Geometry check sheet. Reference: the model listing, model coordinates, mm. Round coordinates to 2 decimals unless told otherwise and drop trailing zeros. Write each loop counter-clockwise with the first axis right and the second up, starting at its lowest first coordinate (ties: lowest second). Pieces come first, ordered by that corner, then holes.
Item 1: Depth check by flat-ended pin: P1, Ø6.5, axis at x = -259.97, y = -86.86, coming from the -Z side; P2, Ø2, axis at y = -197.5, z = -4, coming from the -X side; P3, Ø2, axis at y = 218, z = -1, coming from the +X side. Enter the tip coordinate at first touch or a pass-through.
Item 2: Cross-section at A-A (z = -2.5). Enter the section's corners in (x, y).
Item 3: Draft check along X on faces 1 (the face through (288.249, 120.906, -5.706)), 2 (the face through (-28, 27, 0)). Enter one of: pulls with the +X half, pulls with the -X half, needs draft (parallel to the pull), parting line crosses it, or undercut.
Item 4: Scan lines: probe 1 along Y at (x, z) = (174.5, -4); probe 2 along X at (y, z) = (16, -5.5); probe 3 along X at (y, z) = (157, -2.5). Record each from-to range of solid material in increasing order.
from build123d import *

# Parameters (mm, degrees)
F0_R     = 327.025
F1_DEPTH = 6.35
F3_D     = 7.9375
F5_D     = 7.9375
F6_R     = 5.08


with BuildPart() as f1:
    # F0 (on Top) → F1 (new body)
    with BuildSketch(Plane.XY):
        with Locations((-23.674974, 22.676632)):
            Circle(F0_R)
    extrude(amount=-F1_DEPTH)

    # F3 (through all)
    with Locations(Plane.XY):
        with Locations((-259.972523, 22.676632), (209.927477, 22.676632)):
            Hole(F3_D / 2)

    # F5 (through all)
    with Locations(Plane.XY):
        with Locations((-259.972523, 132.214132), (-259.972523, -86.860868), (209.927477, -86.860868), (209.927477, 132.214132)):
            Hole(F5_D / 2)

    # F6
    f6_edges = [f1.edges().sort_by_distance(p)[0] for p in [
        (-350.699974, 22.676632, 0),
    ]]
    fillet(f6_edges, radius=F6_R)


solid = f1.part
Resolved:
1. P1: passes through
1. P2: stops at x = -266.26
1. P3: stops at x = 237.56
2. outline: circle Ø652.64 at (-23.67, 22.68); hole circle Ø7.94 at (-259.97, -86.86); hole circle Ø7.94 at (-259.97, 22.68); hole circle Ø7.94 at (-259.97, 132.21); hole circle Ø7.94 at (209.93, -86.86); hole circle Ø7.94 at (209.93, 22.68); hole circle Ø7.94 at (209.93, 132.21)
3. face 1: parting line crosses it
3. face 2: needs draft
4. probe 1: y = -237.32 to 282.67
4. probe 2: x = -350.63 to 303.28
4. probe 3: x = -321.07 to 273.72
